Input: dimensioned drawing with shaded views. Units: mm. Origin: part minimum x, y, z. Coordinates: 2 decimals unless noted, no trailing zeros. Write each loop counter-clockwise with the first axis right and the second up, starting at its lowest first coordinate (ties: lowest second). Pieces come first, ordered by that corner, then holes. Notation, with made-up numbers: M 44.5,-22 L 72.5,-22 A17 cw 72.5,7 Z; hole C 17,54.5 d6. An arc over 180 degrees is marked long. Write each question's results on one line, items separated by ' | '. Start each with the question number.
1. Ray query, probe 1 along X at (y, z) = (3, 4.25); probe 2 along X at (y, z) = (8.5, 5.75) (1 decimal); probe 3 along X at (y, z) = (10.25, 6) (1 decimal). Return the intervals inside material, ascending.
2. First-contact query: pin 1 (4 mm diameter, centred on x = 34, z = 7.5, fed in from +Y); pin 2 (1.3 mm diameter, centred on y = 4.5, z = 8, fed in from -X); pin 3 (1.9 mm diameter, centred on x = 40, z = 4.5, fed in from +Y) (1 decimal); pin 4 (4 mm diameter, centred on x = 7.5, z = 6, fed in from +Y). Flat tips, straight axial feed; report the tip coordinate or a pass-through.
3. Section query B-B, the plane x = 43. Output: boundary loops of the cut face in (y, z) (1 decimal), and give its area (3 significant figures).
4. Section query D-D, the plane x = 25. Output: boundary loops of the cut face in (y, z), and give its area (3 significant figures).
5. Section query A-A, the plane y = 3.75. Output: boundary loops of the cut face in (x, z), and give its area (3 significant figures).
6. Pull-direction query (X, two-part tool) for the marked faces 1, 2, 3 and 4; classes: +X half, -X half, draft (parallel to the pull), parting line (faces both ways), or undercut.
7. Section query C-C, the plane z = 10.5. Count the separate pieces of the cut face and the enclosed holes in it.
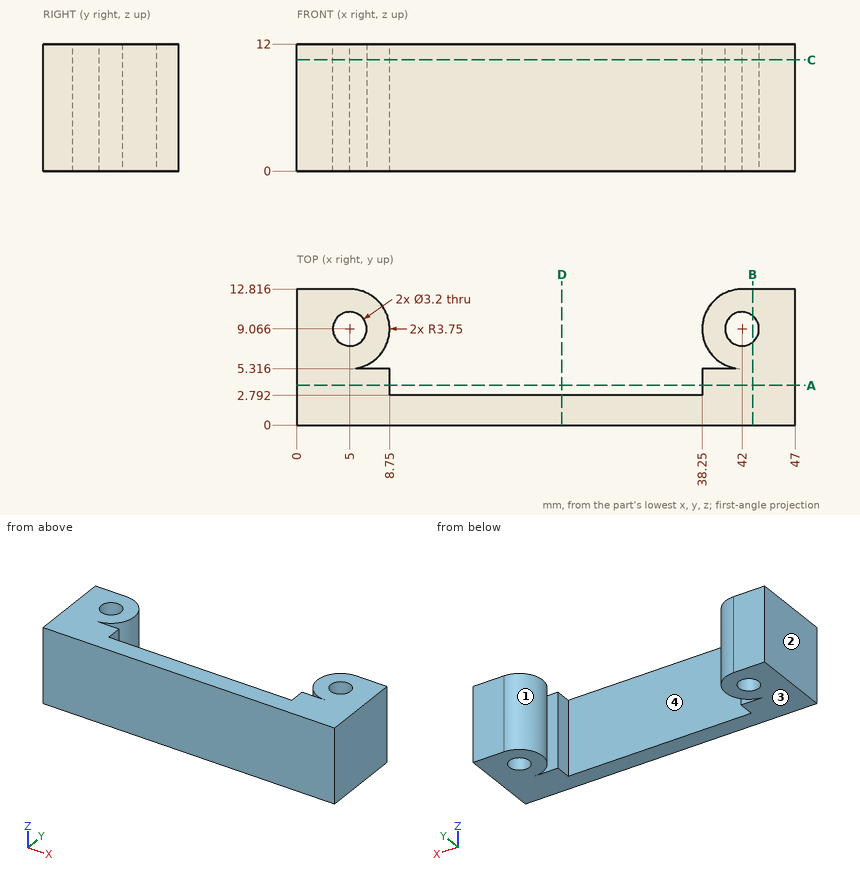
Answer:
1) probe 1: 0 to 8.75, 38.25 to 47 | probe 2: 0 to 3.5, 6.5 to 8.7, 38.3 to 40.5, 43.5 to 47 | probe 3: 0 to 3.9, 6.1 to 8.6, 38.4 to 40.9, 43.1 to 47
2) pin 1: y = 2.79 | pin 2: x = 0 | pin 3: y = 12.7 | pin 4: y = 12.78
3) outline: M 0,0 L 7.8,0 L 7.8,12 L 0,12 Z; M 10.3,0 L 12.8,0 L 12.8,12 L 10.3,12 Z | area: 124 mm^2
4) outline: M 0,0 L 2.79,0 L 2.79,12 L 0,12 Z | area: 33.5 mm^2
5) outline: M 0,0 L 8.75,0 L 8.75,12 L 0,12 Z; M 38.25,0 L 47,0 L 47,12 L 38.25,12 Z | area: 210 mm^2
6) face 1: undercut | face 2: -X half | face 3: draft | face 4: undercut
7) separate pieces: 1 | enclosed holes: 2
